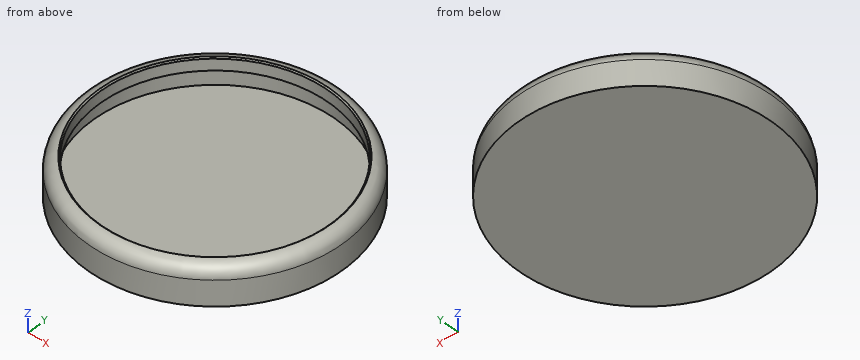
```python
from build123d import *

# Parameters (mm, degrees)
FILLET_R     = 10
SKETCH001_R  = 90
POCKET_DEPTH = 25
CHAMFER_SIZE = 1


with BuildPart() as part:
    # Sketch → Revolution (revolve)
    with BuildSketch(Plane.XZ):
        Polygon((0, 0), (-100, 0), (-100, 30), (0, 30), (0, 20), (-95, 20), (-95, 5), (0, 5), align=None)
    revolve(axis=Axis((0, 0, 0), (0, 0, 1)))

    # Fillet
    fillet_edges = [part.edges().sort_by_distance(p)[0] for p in [
        (100, 0, 30),
    ]]
    fillet(fillet_edges, radius=FILLET_R)

    # Sketch001 → Pocket (cut)
    with BuildSketch(Plane(origin=(0, 0, 30), x_dir=(-1, 0, 0), z_dir=(0, 0, 1))):
        Circle(SKETCH001_R)
    extrude(amount=-POCKET_DEPTH, mode=Mode.SUBTRACT)

    # Chamfer
    chamfer_edges = [part.edges().sort_by_distance(p)[0] for p in [
        (90, 0, 30),
    ]]
    chamfer(chamfer_edges, length=CHAMFER_SIZE)


solid = part.part
```
Source: CAD feature listing. Evaluate the final solid. Frame: model axes, mm. Give positions to 0.01 mm unless a question says otherwise; leave off trailing zeros. Write each loop counter-clockwise with the first axis right and the second up, starting at its lowest first coordinate (ties: lowest second). Pieces come first, ordered by that corner, then holes. Notation, with made-up numbers: (22, -23.5) - (72, -23.5) arc R31 ccw to (72, 3.5) - close; hole circle Ø1 at (-39.75, 1). An arc over 180 degrees is marked (long way). One line per item, written item: value. Start each with the question number.
Q1. Section query B-B, the plane z = 23. Return the cut outline in (x, y), then the cut area to 3 significant figures.
Q2. First-contact query: pin 1 Ø12 at (x, y) = (55, 19) entering from +Z; pin 2 Ø4 at (y, z) = (-11.5, 15.5) entering from +X; pin 3 Ø6 at (y, z) = (16, 4.5) entering from -X. Flat tips, straight axial feed; report the tip coordinate or a pass-through.
Q3. Section query A-A, the plane z = 7.5. Return the cut outline in (x, y), then the cut area to 3 significant figures.
Q4. Material intervals for probe 1 along X at (y, z) = (0, 12); probe 2 along Z at (x, y) = (56, 35.5), sorted ascending. Write a range as from..to.
Answer:
1. outline: circle Ø199.08 at (0, 0); hole circle Ø180 at (0, 0)
1. area: 5,680 mm2
2. pin 1: stops at z = 5
2. pin 2: stops at x = 99.55
2. pin 3: stops at x = -99.15
3. outline: circle Ø200 at (0, 0); hole circle Ø190 at (0, 0)
3. area: 3,060 mm2
4. probe 1: x = -100..-95, 95..100
4. probe 2: z = 0..5
